Build history of the part. All positions in model axes, mm. A direction names the side the tool comes from. Coordinates: 2 decimals unless noted, no trailing zeros. Order: outer loops, then holes, each group sorted by start corner. A loop starts at its lowest first (then second) coordinate and runs counter-clockwise, first axis right, second up. Notation, with made-up numbers: (21.25, 45) - (44.25, 45) arc R31 ccw to (44.25, 78) - close; hole circle Ø8 at (54, 50). An arc over 180 degrees is marked (long way). Write each question's results on one line, items separated by ' | '. Start each with the question number.
from build123d import *

# Parameters (mm, degrees)
F0_R     = 50.8
F0_R_2   = 40
F1_DEPTH = 50
F2_R     = 70.8
F2_R_2   = 3.3
F2_R_3   = 50.8
F3_DEPTH = 5


with BuildPart() as f1:
    # F0 (on Top) → F1 (new body)
    with BuildSketch(Plane.XY):
        Circle(F0_R)
        Circle(F0_R_2, mode=Mode.SUBTRACT)
    extrude(amount=F1_DEPTH)

    # F2 (on Top) → F3 (join)
    with BuildSketch(Plane.XY):
        Circle(F2_R)
        with Locations((-42.992092, -42.992092)):
            Circle(F2_R_2, mode=Mode.SUBTRACT)
        with Locations((0, -60.8)):
            Circle(F2_R_2, mode=Mode.SUBTRACT)
        with Locations((42.992092, -42.992092)):
            Circle(F2_R_2, mode=Mode.SUBTRACT)
        with Locations((-60.8, 0)):
            Circle(F2_R_2, mode=Mode.SUBTRACT)
        with Locations((-42.992092, 42.992092)):
            Circle(F2_R_2, mode=Mode.SUBTRACT)
        Circle(F2_R_3, mode=Mode.SUBTRACT)
        with Locations((60.8, 0)):
            Circle(F2_R_2, mode=Mode.SUBTRACT)
        with Locations((0, 60.8)):
            Circle(F2_R_2, mode=Mode.SUBTRACT)
        with Locations((42.992092, 42.992092)):
            Circle(F2_R_2, mode=Mode.SUBTRACT)
    extrude(amount=F3_DEPTH)


solid = f1.part
Item 1: Probe probe 1 along Y at (x, z) = (0, 1); probe 2 along Y at (x, z) = (0, 27); probe 3 along Z at (x, y) = (-48, -46). List the from-to ranges inside material, lowest first.
Item 2: Slice it at B-B (y = -25). Write the cut outline in (x, z), then the cut area to 3 significant figures.
Item 3: Slice it at C-C (x = 19). Write the cut outline in (y, z), then the cut area to 3 significant figures.
Item 4: Slice it at D-D (z = 19). Write the cut outline in (x, y), then the cut area to 3 significant figures.
Item 5: Slice it at A-A (x = 0). Write the cut outline in (y, z), then the cut area to 3 significant figures.
Item 6: Flat gauge pins, fed straight in: P1, Ø5, axis at x = 28.5, z = 29, coming from the -Y side; P2, Ø2, axis at y = 19, z = 20.5, coming from the -X side; P3, Ø5.5, axis at x = -60.8, y = 0, coming from the +Z side; P4, Ø12, axis at y = -14.5, z = 34, coming from the +X side. Where does each tip first touch, or does it go through?
Item 7: Pull direction Y, two halves, no side cores. Call faces 1 (the cylindrical face through (-11.012, -49.592, 27.185)), 2 (the flat face through (30, -30, 0)), 3 (the cylindrical face through (-57.65, 0.99, 2.46)), 4 (the cylindrical face through (1.774, 63.583, 2.465)): released by +Y, released by -Y, zero draft, split by the parting line, or undercut.
Item 8: Which spindle directions (+Z, -Z, +X, -X, +Y, -Y) get a long thin tool onto all of the face, cutting with end or side? Do faces 5 (the cylindrical face through (57.5, 0.1, 2.5)), 6 (the flat face through (0, -52, 5)). Say none if no direction does.
Resolved:
1) probe 1: -70.8 to -64.1, -57.5 to -40, 40 to 57.5, 64.1 to 70.8 | probe 2: -50.8 to -40, 40 to 50.8 | probe 3: 0 to 5
2) outline: (-66.24, 0) - (-31.22, 0) - (-31.22, 50) - (-44.22, 50) - (-44.22, 5) - (-66.24, 5) - close; (31.22, 0) - (66.24, 0) - (66.24, 5) - (44.22, 5) - (44.22, 50) - (31.22, 50) - close | area: 1,520 mm^2
3) outline: (-68.2, 0) - (-35.2, 0) - (-35.2, 50) - (-47.11, 50) - (-47.11, 5) - (-68.2, 5) - close; (35.2, 0) - (68.2, 0) - (68.2, 5) - (47.11, 5) - (47.11, 50) - (35.2, 50) - close | area: 1,400 mm^2
4) outline: circle Ø101.6 at (0, 0); hole circle Ø80 at (0, 0) | area: 3,080 mm^2
5) outline: (-70.8, 0) - (-64.1, 0) - (-64.1, 5) - (-70.8, 5) - close; (-57.5, 0) - (-40, 0) - (-40, 50) - (-50.8, 50) - (-50.8, 5) - (-57.5, 5) - close; (40, 0) - (57.5, 0) - (57.5, 5) - (50.8, 5) - (50.8, 50) - (40, 50) - close; (64.1, 0) - (70.8, 0) - (70.8, 5) - (64.1, 5) - close | area: 1,210 mm^2
6) P1: y = -43.64 | P2: x = -47.5 | P3: through | P4: x = 50.08
7) face 1: split by the parting line | face 2: zero draft | face 3: undercut | face 4: undercut
8) face 5: +Z, -Z | face 6: +Z
